```python
from build123d import *

# Parameters (mm, degrees)
PAD_DEPTH            = 50
POCKET_DEPTH         = 47.5
PAD001_DEPTH         = 3
POCKET001_DEPTH      = 3.4
POCKET002_DEPTH      = 47.501
POCKET002_DEPTH_BACK = -47.501
POCKET003_DEPTH      = 75.001
POCKET003_DEPTH_BACK = -75.001
SKETCH009_W          = 9
SKETCH009_H          = 46
SKETCH009_W_2        = 118
SKETCH009_H_2        = 5.5
POCKET004_DEPTH      = 1.5


with BuildPart() as part:
    # Sketch003 → Pad (new body)
    with BuildSketch(Plane.XY):
        with BuildLine():
            Line((-72, 47.5), (72, 47.5))
            ThreePointArc((75, 44.5), (74.12132, 46.62132), (72, 47.5))
            Line((75, 44.5), (75, -44.5))
            ThreePointArc((72, -47.5), (74.12132, -46.62132), (75, -44.5))
            Line((72, -47.5), (-72, -47.5))
            ThreePointArc((-75, -44.5), (-74.12132, -46.62132), (-72, -47.5))
            Line((-75, -44.5), (-75, 44.5))
            ThreePointArc((-72, 47.5), (-74.12132, 46.62132), (-75, 44.5))
        make_face()
    extrude(amount=PAD_DEPTH)

    # Sketch004 → Pocket (cut)
    with BuildSketch(Plane.XY.offset(50)):
        with BuildLine():
            Line((-72, 32.5), (-72, -32.5))
            ThreePointArc((-72, -32.5), (-71.707107, -33.207107), (-71, -33.5))
            Line((-71, -33.5), (-68, -33.5))
            ThreePointArc((-67, -34.5), (-67.292893, -33.792893), (-68, -33.5))
            Line((-67, -34.5), (-67, -37.5))
            ThreePointArc((-67, -37.5), (-66.414214, -38.914214), (-65, -39.5))
            Line((-65, -39.5), (-62, -39.5))
            ThreePointArc((-61, -40.5), (-61.292893, -39.792893), (-62, -39.5))
            Line((-61, -40.5), (-61, -43.5))
            ThreePointArc((-61, -43.5), (-60.707107, -44.207107), (-60, -44.5))
            Line((-60, -44.5), (60, -44.5))
            ThreePointArc((60, -44.5), (60.707107, -44.207107), (61, -43.5))
            Line((61, -43.5), (61, -40.5))
            ThreePointArc((62, -39.5), (61.292893, -39.792893), (61, -40.5))
            Line((62, -39.5), (65, -39.5))
            ThreePointArc((65, -39.5), (66.414214, -38.914214), (67, -37.5))
            Line((67, -37.5), (67, -34.5))
            ThreePointArc((68, -33.5), (67.292893, -33.792893), (67, -34.5))
            Line((68, -33.5), (71, -33.5))
            ThreePointArc((71, -33.5), (71.707107, -33.207107), (72, -32.5))
            Line((72, -32.5), (72, 32.5))
            ThreePointArc((72, 32.5), (71.707107, 33.207107), (71, 33.5))
            Line((71, 33.5), (68, 33.5))
            ThreePointArc((67, 34.5), (67.292893, 33.792893), (68, 33.5))
            Line((67, 34.5), (67, 37.5))
            ThreePointArc((67, 37.5), (66.414214, 38.914214), (65, 39.5))
            Line((65, 39.5), (62, 39.5))
            ThreePointArc((61, 40.5), (61.292893, 39.792893), (62, 39.5))
            Line((61, 40.5), (61, 43.5))
            ThreePointArc((61, 43.5), (60.707107, 44.207107), (60, 44.5))
            Line((60, 44.5), (-60, 44.5))
            ThreePointArc((-60, 44.5), (-60.707107, 44.207107), (-61, 43.5))
            Line((-61, 43.5), (-61, 40.5))
            ThreePointArc((-62, 39.5), (-61.292893, 39.792893), (-61, 40.5))
            Line((-62, 39.5), (-65, 39.5))
            ThreePointArc((-65, 39.5), (-66.414214, 38.914214), (-67, 37.5))
            Line((-67, 37.5), (-67, 34.5))
            ThreePointArc((-68, 33.5), (-67.292893, 33.792893), (-67, 34.5))
            Line((-68, 33.5), (-71, 33.5))
            ThreePointArc((-71, 33.5), (-71.707107, 33.207107), (-72, 32.5))
        make_face()
    extrude(amount=-POCKET_DEPTH, mode=Mode.SUBTRACT)

    # Sketch005 → Pad001 (join)
    with BuildSketch(Plane.XY.offset(50)):
        with BuildLine():
            Line((-70, 42.5), (-70, 36.5))
            Line((-70, 36.5), (-72, 36.5))
            Line((-72, 36.5), (-72, 43.5))
            ThreePointArc((-71, 44.5), (-71.707107, 44.207107), (-72, 43.5))
            Line((-71, 44.5), (-64, 44.5))
            Line((-64, 44.5), (-64, 42.5))
            Line((-64, 42.5), (-70, 42.5))
        make_face()
        with BuildLine():
            Line((64, 42.5), (70, 42.5))
            Line((70, 42.5), (70, 36.5))
            Line((70, 36.5), (72, 36.5))
            Line((72, 43.5), (72, 36.5))
            ThreePointArc((72, 43.5), (71.707107, 44.207107), (71, 44.5))
            Line((64, 44.5), (71, 44.5))
            Line((64, 44.5), (64, 42.5))
        make_face()
        with BuildLine():
            Line((72, -36.5), (70, -36.5))
            Line((70, -36.5), (70, -42.5))
            Line((70, -42.5), (64, -42.5))
            Line((64, -42.5), (64, -44.5))
            Line((64, -44.5), (71, -44.5))
            ThreePointArc((71, -44.5), (71.707107, -44.207107), (72, -43.5))
            Line((72, -43.5), (72, -36.5))
        make_face()
        with BuildLine():
            Line((-70, -36.5), (-70, -42.5))
            Line((-70, -42.5), (-64, -42.5))
            Line((-64, -42.5), (-64, -44.5))
            Line((-64, -44.5), (-71, -44.5))
            ThreePointArc((-72, -43.5), (-71.707107, -44.207107), (-71, -44.5))
            Line((-72, -43.5), (-72, -36.5))
            Line((-72, -36.5), (-70, -36.5))
        make_face()
    extrude(amount=PAD001_DEPTH)

    # Sketch006 → Pocket001 (cut)
    with BuildSketch(Plane.XY):
        with BuildLine():
            Line((-72.4, 44.9), (-72.4, 36.1))
            Line((-72.4, 36.1), (-69.6, 36.1))
            Line((-69.6, 36.1), (-69.6, 41.1))
            ThreePointArc((-68.6, 42.1), (-69.307107, 41.807107), (-69.6, 41.1))
            Line((-68.6, 42.1), (-63.6, 42.1))
            Line((-63.6, 42.1), (-63.6, 44.9))
            Line((-63.6, 44.9), (-72.4, 44.9))
        make_face()
        with BuildLine():
            Line((63.6, 44.9), (72.4, 44.9))
            Line((72.4, 44.9), (72.4, 36.1))
            Line((72.4, 36.1), (69.6, 36.1))
            Line((69.6, 36.1), (69.6, 41.1))
            ThreePointArc((69.6, 41.1), (69.307107, 41.807107), (68.6, 42.1))
            Line((68.6, 42.1), (63.6, 42.1))
            Line((63.6, 42.1), (63.6, 44.9))
        make_face()
        with BuildLine():
            Line((69.6, -36.1), (72.4, -36.1))
            Line((72.4, -36.1), (72.4, -44.9))
            Line((72.4, -44.9), (63.6, -44.9))
            Line((63.6, -44.9), (63.6, -42.1))
            Line((63.6, -42.1), (68.6, -42.1))
            ThreePointArc((68.6, -42.1), (69.307107, -41.807107), (69.6, -41.1))
            Line((69.6, -41.1), (69.6, -36.1))
        make_face()
        with BuildLine():
            Line((-63.6, -42.1), (-63.6, -44.9))
            Line((-63.6, -44.9), (-72.4, -44.9))
            Line((-72.4, -44.9), (-72.4, -36.1))
            Line((-72.4, -36.1), (-69.6, -36.1))
            Line((-69.6, -36.1), (-69.6, -41.1))
            ThreePointArc((-69.6, -41.1), (-69.307107, -41.807107), (-68.6, -42.1))
            Line((-68.6, -42.1), (-63.6, -42.1))
        make_face()
    extrude(amount=POCKET001_DEPTH, mode=Mode.SUBTRACT)

    # Sketch007 → Pocket002 (cut, two sides)
    with BuildSketch(Plane.XZ) as pocket002_sk:
        with BuildLine():
            Line((-45, 53), (-45, 47))
            ThreePointArc((-45, 47), (-42.803301, 41.696699), (-37.5, 39.5))
            Line((-37.5, 39.5), (37.5, 39.5))
            ThreePointArc((37.5, 39.5), (42.803301, 41.696699), (45, 47))
            Line((45, 47), (45, 50))
            Line((45, 53), (45, 50))
            Line((-45, 53), (45, 53))
        make_face()
    extrude(amount=-POCKET002_DEPTH, mode=Mode.SUBTRACT)
    extrude(pocket002_sk.sketch, amount=-POCKET002_DEPTH_BACK, mode=Mode.SUBTRACT)

    # Sketch008 → Pocket003 (cut, two sides)
    with BuildSketch(Plane.YZ) as pocket003_sk:
        with BuildLine():
            ThreePointArc((-12.5, 43), (-19.5, 36), (-12.5, 29))
            Line((-12.5, 29), (12.5, 29))
            ThreePointArc((12.5, 29), (19.5, 36), (12.5, 43))
            Line((12.5, 43), (-12.5, 43))
        make_face()
    extrude(amount=-POCKET003_DEPTH, mode=Mode.SUBTRACT)
    extrude(pocket003_sk.sketch, amount=-POCKET003_DEPTH_BACK, mode=Mode.SUBTRACT)

    # Sketch009 → Pocket004 (cut)
    with BuildSketch(Plane.XZ.offset(47.5)):
        with Locations((-66.5, 25)):
            Rectangle(SKETCH009_W, SKETCH009_H)
        with Locations((66.5, 25)):
            Rectangle(SKETCH009_W, SKETCH009_H)
        with BuildLine():
            ThreePointArc((-48, 47), (-44.924621, 39.575379), (-37.5, 36.5))
            Line((-37.5, 36.5), (37.5, 36.5))
            ThreePointArc((37.5, 36.5), (44.924621, 39.575379), (48, 47))
            Line((48, 47), (48, 48))
            Line((48, 48), (59, 48))
            Line((59, 48), (59, 32.5))
            Line((59, 32.5), (-59, 32.5))
            Line((-59, 32.5), (-59, 48))
            Line((-59, 48), (-48, 48))
            Line((-48, 48), (-48, 47))
        make_face()
        with Locations((0, 27.75)):
            Rectangle(SKETCH009_W_2, SKETCH009_H_2)
    pocket004 = extrude(amount=-POCKET004_DEPTH, mode=Mode.SUBTRACT)

    # Mirrored: Pocket004 across XZ
    add(pocket004.mirror(Plane.XZ), mode=Mode.SUBTRACT)


solid = part.part
```
Read the model definition and answer for the solid it produces. Units are mm, in the model's axes. A direction names the side the tool comes from. Coordinates: 2 decimals unless noted, no trailing zeros. Order: outer loops, then holes, each group sorted by start corner. A loop starts at its lowest first (then second) coordinate and runs counter-clockwise, first axis right, second up. Notation, with made-up numbers: (-36, 75.5) - (-2, 75.5) arc R23 cw to (-2, 106.5) - close; hole circle Ø9 at (38.25, -0.5). An arc over 180 degrees is marked (long way). Answer as a JSON object with one key per item and string values. Group by question number.
Item 1: The mould has two halves that part along Y. Classify faces 1 (the face through (70, -43, 53)), 2 (the face through (1, 44.5, 21)), 3 (the face through (-69.6, -39, 2)), 4 (the face through (-1, 46, 28)): +Y half, -Y half, draft (parallel to the pull), parting line (faces both ways), or undercut.
Item 2: Consider probe 1 along Y at (x, z) = (49, 16.5); probe 2 along X at (y, z) = (14, 18.5); probe 3 along Y at (x, z) = (-36.5, 26). Determine where each line is inside the solid, lowest interval first. Write a range as from..to.
Item 3: Section B-B (z = 41) is taken. State how many separate pieces and enclosed holes the cut face has, plus the area to 3 significant figures.
Item 4: Section A-A (x = -16) is taken. Give the vertices of the cut face in (y, z).
Item 5: Flat-ended cylindrical pins translate along their axes: P1, Ø1.6, axis at x = -71.5, z = 51, coming from the +Y side; P2, Ø2.5, axis at x = 67.5, z = 51.5, coming from the -Y side; P3, Ø6, axis at x = 29.5, z = 25.5, coming from the -Y side; P4, Ø6, axis at x = -17.5, y = -28, coming from the +Z side. Find the tip coordinate at first contact, or state that the pin passes through.
Item 6: Section C-C (x = -42) is taken. Give the vertices of the cut face in (y, z), plus the area to 3 significant figures.
Item 7: A tool of negligible diameter and unlimited length cuts with its end or side. For faces 5 (the face through (-69.6, 39, 2)), 6 (the face through (-67, -44.5, 51)), 7 (the face through (-42.861, -45.979, 41.755)), 8 (the face through (73.48, -19.5, 36.15)), from which of +Z, -Z, +X, -X, +Y, -Y can it reach the whole face along a straight path? Write none if from no direction.
Results are:
{
 "1": {"face 1": "draft", "face 2": "undercut", "face 3": "undercut", "face 4": "+Y half"},
 "2": {"probe 1": "y = -47.5..-44.5, 44.5..47.5", "probe 2": "x = -75..-72, 72..75", "probe 3": "y = -46..-44.5, 44.5..46"},
 "3": {"separate pieces": "4", "enclosed holes": "0", "area": "926 mm^2"},
 "4": {"outline": "(-47.5, 0) - (47.5, 0) - (47.5, 25) - (46, 25) - (46, 30.5) - (47.5, 30.5) - (47.5, 32.5) - (46, 32.5) - (46, 36.5) - (47.5, 36.5) - (47.5, 39.5) - (44.5, 39.5) - (44.5, 2.5) - (-44.5, 2.5) - (-44.5, 39.5) - (-47.5, 39.5) - (-47.5, 36.5) - (-46, 36.5) - (-46, 32.5) - (-47.5, 32.5) - (-47.5, 30.5) - (-46, 30.5) - (-46, 25) - (-47.5, 25) - close"},
 "5": {"P1": "stops at y = 44.5", "P2": "stops at y = -44.5", "P3": "stops at y = -47.5", "P4": "stops at z = 2.5"},
 "6": {"outline": "(-47.5, 0) - (47.5, 0) - (47.5, 25) - (46, 25) - (46, 30.5) - (47.5, 30.5) - (47.5, 32.5) - (46, 32.5) - (46, 37.51) - (47.5, 37.51) - (47.5, 41) - (44.5, 41) - (44.5, 2.5) - (-44.5, 2.5) - (-44.5, 41) - (-47.5, 41) - (-47.5, 37.51) - (-46, 37.51) - (-46, 32.5) - (-47.5, 32.5) - (-47.5, 30.5) - (-46, 30.5) - (-46, 25) - (-47.5, 25) - close", "area": "437 mm^2"},
 "7": {"face 5": "-Z", "face 6": "+Z, +X, -X, -Y", "face 7": "+Z, +Y, -Y", "face 8": "+X, -X"}
}
